The listing builds one solid part. Answer for the finished solid, in the listing's coordinates (mm). Face numbers are marked on the shaded views. A direction names the side the tool comes from. Give positions to 0.01 mm unless a question says otherwise; leave off trailing zeros. Write each loop counter-clockwise with the first axis right and the second up, starting at its lowest first coordinate (ties: lowest second). Pieces come first, ordered by that corner, then holes. Notation, with made-up numbers: (55, -10) - (78, -10) arc R21 ccw to (78, 8) - close; hole circle Ø11 at (39, 3.5). An arc over 180 degrees is marked (long way). One line per item, written item: value. Start each with the question number.
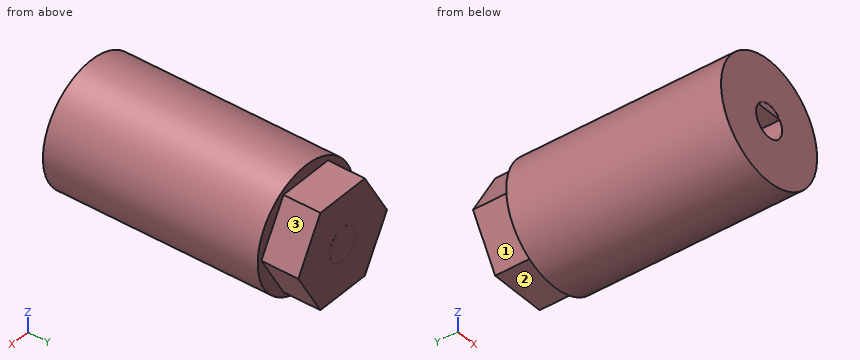
Autodesk Inventor part; units mm, degrees
ref_plane "YZ Plane" through (0, 0, 0) normal (1, 0, 0) x (0, 1, 0)
ref_plane "XZ Plane" through (0, 0, 0) normal (0, 1, 0) x (-1, 0, 0)
ref_plane "XY Plane" through (0, 0, 0) normal (0, 0, 1) x (1, 0, 0)
sketch "Sketch1" plane through (0, 0, 0) normal (0, 1, 0) x (-1, 0, 0)
  line L0 (-3.4641, -6) -> (-6.9282, 0)
  line L1 (-6.9282, 0) -> (-3.4641, 6)
  line L2 (-3.4641, 6) -> (3.4641, 6)
  line L3 (3.4641, 6) -> (6.9282, 0)
  line L4 (6.9282, 0) -> (3.4641, -6)
  line L5 (3.4641, -6) -> (-3.4641, -6)
  line L6 (10.5, 0) -> (-10.5, 0)
  line L7 (0, -10.5) -> (0, 10.5)
  circle A0 centre (0, 0) radius 2
  arc A1 (0.4459, -1.9497) -> (0.4459, -1.9497) centre (0, 0) ccw
  line L8 (1.64, 1.1447) -> (-1.64, 1.1447)
  circle A2 centre (0, 0) radius 2.025
  circle A3 centre (0, 0) radius 7.5
  dimension "d2" = 4
  dimension "d6" = 4.05
  dimension "d33" = 15
  dimension "d36" = 3.28
  dimension "d37" = 12
extrude "Extrusion1" add sketch "Sketch1" along normal blind 4.57 contours L0 L6 A2 L7 L5 | L1 L2 L7 A2 L6 | L7 A2 L6 L4 L5 | L6 A0 L7 A2 | L7 A0 L6 A2 | L2 L3 L6 A2 L7 picked at (-1.8669, -0.7323) picked at (1.9162, -0.5914)
extrude "Extrusion6" add sketch "Sketch1" along normal blind 4.572 contours A2 L7 A0 L6 | L6 A0 L7 A2 | L7 A0 L6 A2 | A0 L8 L7 L6 | L6 L7 A0 | A2 L6 A0 L7 | L7 L6 A0 | L7 L8 A0 L6 | A0 L7 L8 | A0 L8 L7
extrude "Extrusion11" add sketch "Sketch1" against normal blind 17.8 contours A2 L7 A0 L6 | L6 A0 L7 A2 | L7 A0 L6 A2 | A0 L8 L7 L6 | L6 L7 A0 | A2 L6 A0 L7 | L7 L6 A0 | L7 L8 A0 L6 | A0 L7 L8 | A0 L8 L7
extrude "Extrusion12" add sketch "Sketch1" against normal blind 26.6 contours A2 L7 A0 L6 | A2 L6 A0 L7 | A0 L7 L8 | A0 L8 L7 picked at (-1.5145, 1.3032) picked at (1.5145, 1.3032)
extrude "Extrusion13" add sketch "Sketch1" against normal blind 26.6 contours L5 L7 A3 L6 L0 | L0 L6 A2 L7 L5 | L6 A3 L7 L2 L1 | L1 L2 L7 A2 L6 | L7 A2 L6 L4 L5 | L5 L4 L6 A3 L7 | L7 A3 L6 L3 L2 | L2 L3 L6 A2 L7
properties part number "wheel connector"
Item 1: Straight lines are drawn through the part: line 1 along Y through (x, z) = (-0.5, 3.25); line 2 along Y through (x, z) = (6.5, 1); line 3 along Z through (x, y) = (-0.25, -11.5). For each, find the intervals that lie inside material, in ascending order.
Item 2: Find section D-D on y = -5. Determine the outline of the cut face in (x, z).
Item 3: Each of these flat-tipped pins is pushed along its axis until it touches: pin 1 Ø3 at (y, z) = (-18, -2.5) entering from -X; pin 2 Ø2.5 at (x, y) = (-1, 2) entering from -Z; pin 3 Ø4 at (x, y) = (-3, -4) entering from -Z; pin 4 Ø6.5 at (x, z) = (0, 0) entering from -Y. Where does it stop, or does it pass through?
Item 4: Find section B-B on y = 1. Determine the outline of the cut face in (x, z).
Item 5: For the marked faces 1, 2 and 3, determine the directions among +Z, -Z, +X, -X, +Y, -Y from which every point of the face is accessible in a straight line to the end or side of a thin tool.
Values:
1. line 1: -26.6 to 4.57
1. line 2: -26.6 to 0
1. line 3: -7.5 to 7.5
2. outline: circle Ø15 at (0, 0)
3. pin 1: x = -7.43
3. pin 2: z = -6
3. pin 3: z = -7.43
3. pin 4: y = -26.6
4. outline: (-6.93, 0) - (-3.46, -6) - (3.46, -6) - (6.93, 0) - (3.46, 6) - (-3.46, 6) - close
5. face 1: -Z, -X, +Y
5. face 2: -Z, +X, -X, +Y
5. face 3: +Z, +X, +Y
